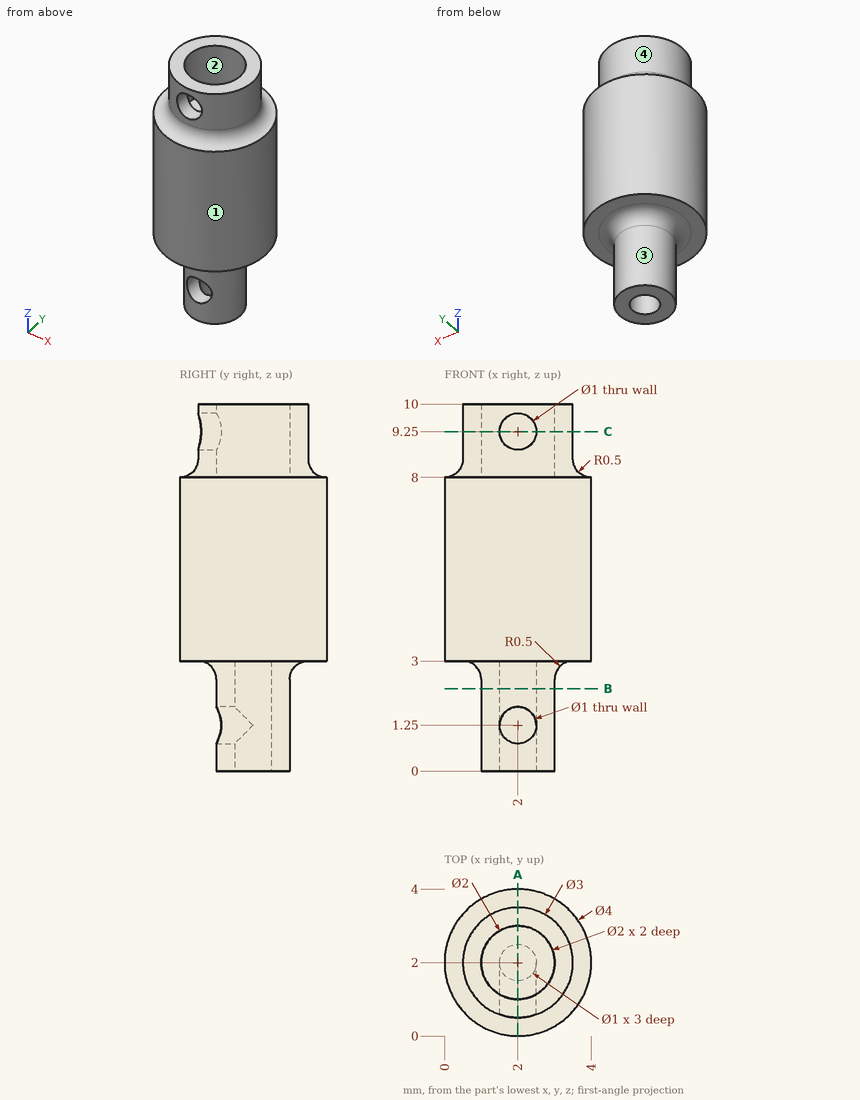
Study the drawing (mm; zero at the part's minimum x, y, z) and answer. A direction names the side the tool comes from. Round coordinates to 2 decimals unless told otherwise and drop trailing zeros. Write each loop counter-clockwise with the first axis right and the second up, starting at its lowest first coordinate (ties: lowest second). Pieces come first, ordered by that corner, then holes. Notation, with made-up numbers: (-35.5, 82.25) -> (-29.5, 82.25) arc R25 ccw to (-29.5, 118.25) -> close; hole circle Ø7 at (-34.5, 69). An arc over 180 degrees is marked (long way). Answer as CSV lines item,"result". Start each with the question number.
(1) Find the intervals of material crossed by probe 1 along X at (y, z) = (2, 0.75); probe 2 along Z at (x, y) = (2.3, 2.5), in increasing order.
(2) Each of these flat-tipped pins is pushed along its axis until it touches: pin 1 (0.8 mm diameter, centred on x = 2, y = 2, fed in from -Z); pin 2 (1.5 mm diameter, centred on y = 0.5, z = 6.5, fed in from -X). Where does it stop, or does it pass through?
(3) The mould has two halves that part along X. Classify the marked faces 1 and 2: +X half, -X half, draft (parallel to the pull), parting line (faces both ways), or undercut.
(4) A tool of negligible diameter and unlimited length cuts with its end or side. For the marked faces 3 and 4, from which of +Z, -Z, +X, -X, +Y, -Y can it reach the whole face along a straight path? Write none if from no direction.
(5) The part is cut by section B-B, the plane z = 2.25. Give the vertices of the cut face in (x, y).
(6) The part is cut by section C-C, the plane z = 9.25. Give the vertices of the cut face in (x, y), then the cut area to 3 significant figures.
(7) The part is cut by section A-A, the plane x = 2. Give the number of separate pieces and of enclosed holes in the cut face, then the cut area to 3 significant figures.
Output values:
1,probe 1,"x = 1 to 1.5, 2.5 to 3"
1,probe 2,"z = 0 to 8"
2,pin 1,"stops at z = 3"
2,pin 2,"stops at x = 0.15"
3,face 1,"parting line"
3,face 2,"undercut"
4,face 3,"-Z"
4,face 4,"+Z"
5,outline,"circle Ø2 at (2, 2); hole circle Ø1 at (2, 2)"
6,outline,"(1.5, 0.59) -> (1.5, 1.13) arc R1 cw (long way) to (2.5, 1.13) -> (2.5, 0.59) arc R1.5 ccw (long way) to start"
6,area,"3.41 mm²"
7,separate pieces,"3"
7,enclosed holes,"0"
7,area,"24.2 mm²"
